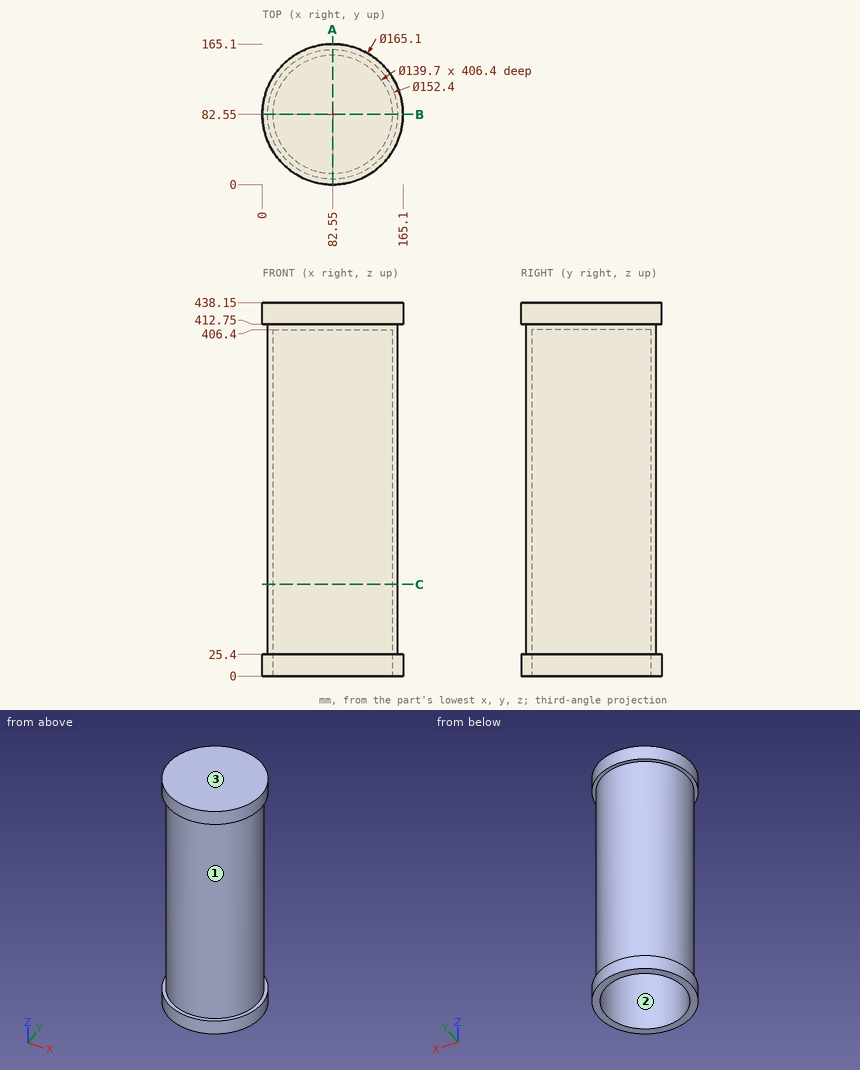
Could you check a few things on this drawing? It's one solid part, dimensions in mm from its lowest x, y, z. Give positions to 0.01 mm unless a question says otherwise; leave off trailing zeros. Write each loop counter-clockwise with the first axis right and the second up, starting at its lowest first coordinate (ties: lowest second). Pieces come first, ordered by that corner, then holes. Notation, with made-up numbers: (3.25, 57) -> (38.25, 57) arc R19 cw to (38.25, 76) -> close; hole circle Ø9 at (85, -18.5). An arc over 180 degrees is marked (long way). Answer as CSV lines item,"result". Start each with the question number.
(1) If we mould it in two halves opening along Z, with no side actions, what happens to the marked faces 1, 2 and 3? For each: +Z half, -Z half, draft (parallel to the pull), parting line (faces both ways), or undercut.
(2) Please list where these lines run through material, in increasing order: line 1 (Y direction, x = 82.55, z = 224); line 2 (X direction, y = 79, z = 262.5).
(3) If we section it at A-A, the plane x = 82.55: Write out the boundary of the cut face in (y, z).
(4) I'm going to push flat-ended pins straight in: pin 1 Ø5 at (x, z) = (44, 339) entering from -Y; pin 2 Ø6 at (x, z) = (139.5, 167.5) entering from +Y; pin 3 Ø10 at (x, y) = (92.5, 141.5) entering from -Z. Where does each tip first touch, or does it pass through?
(5) If we section it at C-C, the plane z = 107.5: Write out the boundary of the cut face in (x, y), and give its area (3 significant figures).
Answer list:
1,face 1,"undercut"
1,face 2,"draft"
1,face 3,"+Z half"
2,line 1,"6.35 to 12.7, 152.4 to 158.75"
2,line 2,"6.43 to 12.79, 152.31 to 158.67"
3,outline,"(0, 0) -> (12.7, 0) -> (12.7, 406.4) -> (152.4, 406.4) -> (152.4, 0) -> (165.1, 0) -> (165.1, 25.4) -> (158.75, 25.4) -> (158.75, 412.75) -> (165.1, 412.75) -> (165.1, 438.15) -> (0, 438.15) -> (0, 412.75) -> (6.35, 412.75) -> (6.35, 25.4) -> (0, 25.4) -> close"
4,pin 1,"y = 15.42"
4,pin 2,"y = 136.36"
4,pin 3,"z = 406.4"
5,outline,"circle Ø152.4 at (82.55, 82.55); hole circle Ø139.7 at (82.55, 82.55)"
5,area,"2,910 mm^2"
